Autodesk Inventor part; units mm, degrees
ref_plane "YZ Plane" through (0, 0, 0) normal (1, 0, 0) x (0, 1, 0)
ref_plane "XZ Plane" through (0, 0, 0) normal (0, 1, 0) x (-1, 0, 0)
ref_plane "XY Plane" through (0, 0, 0) normal (0, 0, 1) x (1, 0, 0)
sketch "Sketch1" plane through (0, 0, 0) normal (0, 1, 0) x (-1, 0, 0)
  circle A0 centre (0, 0) radius 22.9
  circle A1 centre (0, 0) radius 39.5
  circle A2 centre (0, 0) radius 29
  circle A3 centre (0, -29) radius 2.75
  circle A4 centre (29, 0) radius 2.75
  circle A5 centre (0, 29) radius 2.75
  circle A6 centre (-29, 0) radius 2.75
  circle A7 centre (0, 0) radius 25.4
  line L0 (-29, 12.5) -> (29, 12.5)
  line L1 (29, 12.5) -> (29, -12.5)
  line L2 (29, -12.5) -> (-29, -12.5)
  line L3 (-29, -12.5) -> (-29, 12.5)
  line L4 (-29, 12.5) -> (29, -12.5) construction
  line L5 (29, 12.5) -> (-29, -12.5) construction
  point P0 (19.1875, 12.5)
  point P1 (22.1113, 12.5)
  point P2 (-22.1113, 12.5)
  point P3 (-19.1875, 12.5)
  point P4 (-19.1875, -12.5)
  point P5 (-22.1113, -12.5)
  point P6 (22.1113, -12.5)
  point P7 (19.1875, -12.5)
  dimension "d2" = 58
  dimension "d0" = 45.8
  dimension "d1" = 79
  dimension "d3" = 5.5
  dimension "d6" = 360
  dimension "d10" = 25
extrude "Extrusion1" add sketch "Sketch1" along normal blind 5 contours A0 L2 L0 | A0 L0 A7 L2 | L0 A0 | A0 L0 A7 | L2 A7 A0 | A0 L2 | A0 L2 A7 L0 | L0 A2 A4 L2 A7 | A7 L0 A2 A5 | L2 A2 A3 A7 | A7 L2 A2 A6 L0 | L0 L1 A4 A2 | A2 A4 L1 L2 | A2 A6 L3 L0 | L2 L3 A6 A2 | A1
extrude "Extrusion2" add sketch "Sketch1" along normal blind 47 contours A0 L0 A7 | L2 A7 A0
extrude "Extrusion3" add sketch "Sketch1" along normal blind 38 contours A0 L0 A7 L2 | A0 L2 A7 L0
properties part number "PZT holder"
Can you work these out from the model? Positions are in its coordinate system, mm. A direction names the side the tool comes from. Round coordinates to 2 decimals unless told otherwise and drop trailing zeros. Loops run counter-clockwise (first coordinate to the right, second up) from the corner with the lowest first, then second, coordinate; pieces in that order, holes last. Notation, with made-up numbers: M 57,-11 L 103,-11 A21 cw 103,20 Z; hole C 70.5,58.5 d3. An arc over 180 degrees is marked long. Answer as a JSON object with one key per item and string values. Group by question number.
Q1. On a 3-axis mill with a long thin cutter (end or side, diameter ignored), from which of +Z, -Z, +X, -X, +Y, -Y can I reach the whole of each face in a straight line? I mean faces 5 (the cylindrical face through (22.833, 25.706, 1.756)), 6 (the cylindrical face through (-26.253, 2.465, -0.121)), 7 (the flat face through (21, 42, -12.5)). Say none if no direction works.
Q2. Imagine slicing it at A-A, the plane x = 0. Please give me the cut outline in (y, z), then the cut area to 3 significant figures.
Q3. Imagine slicing it at C-C, the plane z = 0. Please give me the cut outline in (x, y).
Q4. Imagine slicing it at D-D, the plane x = 29. Please give me the cut outline in (y, z), then the cut area to 3 significant figures.
Q5. Please list where these lines run through material, in increasing order: L1, parallel to Z at x = 0, y = 3.55; L2, parallel to Z at x = 0, y = 25; L3, parallel to Y at x = -30.5, z = 17.
Q6. Will these pins go through, and if not, where does the flat tip stop? pin 1 (7 mm diameter, centred on x = 23.5, z = -0.5, fed in from +Y); pin 2 (12 mm diameter, centred on x = 28, z = 5.5, fed in from -Y); pin 3 (2.5 mm diameter, centred on x = 20.5, y = 43, fed in from +Z); pin 4 (3 mm diameter, centred on x = -20, y = 44, fed in from +Z).
Q7. Imagine slicing it at B-B, the plane y = 41. Please give me the cut outline in (x, z).
Q8. We'd pull the mould along Z, two halves only. Please class faces 1 (the flat face through (1, 5, -26)), 2 (the cylindrical face through (0.358, 2.465, -31.727)), 3 (the flat face through (-21, 42, 12.5)), 4 (the cylindrical face through (25.153, 25.706, 3.535)): +Z half, -Z half, draft (parallel to the pull), parting line (faces both ways), or undercut.
Findings:
{
 "1": {"face 5": "+Y", "face 6": "+Y, -Y", "face 7": "+X, -X, +Y"},
 "2": {"outline": "M 0,-39.5 L 5,-39.5 L 5,-31.75 L 0,-31.75 Z; M 0,-26.25 L 5,-26.25 L 5,-25.4 L 47,-25.4 L 47,-22.9 L 5,-22.9 L 5,22.9 L 47,22.9 L 47,25.4 L 5,25.4 L 5,26.25 L 0,26.25 Z; M 0,31.75 L 5,31.75 L 5,39.5 L 0,39.5 Z", "area": "550 mm2"},
 "3": {"outline": "M -39.5,0 L -31.75,0 L -31.75,5 L -39.5,5 Z; M -26.25,0 L 26.25,0 L 26.25,5 L 25.4,5 L 25.4,38 L 22.9,38 L 22.9,5 L -22.9,5 L -22.9,38 L -25.4,38 L -25.4,5 L -26.25,5 Z; M 31.75,0 L 39.5,0 L 39.5,5 L 31.75,5 Z"},
 "4": {"outline": "M 0,-26.82 L 5,-26.82 L 5,-2.75 L 0,-2.75 Z; M 0,2.75 L 5,2.75 L 5,26.82 L 0,26.82 Z", "area": "241 mm2"},
 "5": {"L1": "z = -39.5 to -31.75, -26.25 to 26.25, 31.75 to 39.5", "L2": "z = -25.4 to -22.9, 22.9 to 25.4", "L3": "y = 0 to 5"},
 "6": {"pin 1": "stops at y = 38", "pin 2": "stops at y = 0", "pin 3": "stops at z = 16.57", "pin 4": "stops at z = 17.4"},
 "7": {"outline": "M -22.11,-12.5 A25.4 ccw 22.11,-12.5 L 19.19,-12.5 A22.9 cw -19.19,-12.5 Z; M -22.11,12.5 L -19.19,12.5 A22.9 cw 19.19,12.5 L 22.11,12.5 A25.4 ccw Z"},
 "8": {"face 1": "draft", "face 2": "undercut", "face 3": "undercut", "face 4": "parting line"}
}
